Here's the drawing with two shaded views (mm, measured from the low corner). I have some questions. A direction names the side the tool comes from. Round coordinates to 2 decimals unless told otherwise and drop trailing zeros. Order: outer loops, then holes, each group sorted by start corner. A loop starts at its lowest first (then second) coordinate and runs counter-clockwise, first axis right, second up. Notation, with made-up numbers: (57, 20.5) - (102, 20.5) arc R6 cw to (102, 24.5) - close; hole circle Ø3 at (51, -19.5). An arc over 180 degrees is marked (long way). One line per item, written item: value.
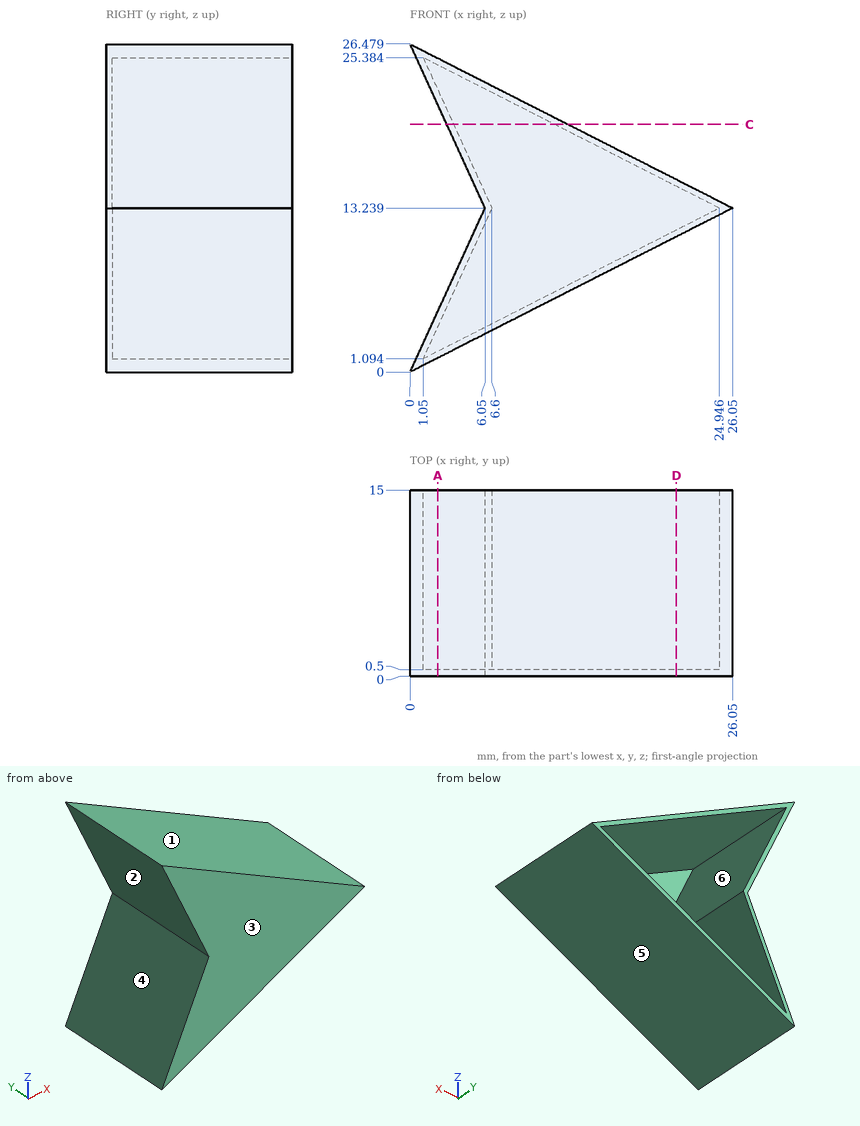
Q1. We'd pull the mould along Z, two halves only. Please class the marked faces 1, 2 and 3: released by +Z, released by -Z, zero draft, split by the parting line, or undercut.
Results list:
face 1: released by +Z
face 2: undercut
face 3: zero draft
Q2. If we section it at C-C, the plane z = 20: Please give me the cut outline in (x, y).
Results list:
outline: (2.96, 0) - (12.75, 0) - (12.75, 15) - (11.64, 15) - (11.64, 0.5) - (3.51, 0.5) - (3.51, 15) - (2.96, 15) - close
Q3. Will these pins go through, and if not, where does the flat tip stop? pin 1 (2 mm diameter, centred on y = 7, z = 17.5, fed in from -X) (1 decimal); pin 2 (5 mm diameter, centred on x = 7.5, y = 9, fed in from -Z); pin 3 (5 mm diameter, centred on y = 12, z = 22.5, fed in from -X) (1 decimal); pin 4 (3 mm diameter, centred on x = 16.5, z = 21, fed in from +Y).
Results list:
pin 1: x = 3.6
pin 2: z = 2.54
pin 3: x = 0.7
pin 4: through
Q4. If I drill on line 1 along Z through (x, y) = (7.75, 7.5); line 2 along X through (y, z) = (6.5, 13.75) (1 decimal); line 3 along Z through (x, y) = (16.25, 14), over which ranges is the centre line in solid material (lowest first)?
Results list:
line 1: 3.94 to 4.5, 21.98 to 22.54
line 2: 5.8 to 6.4, 23.9 to 25
line 3: 8.26 to 8.82, 17.66 to 18.22
Q5. Which directions (+Z, -Z, +X, -X, +Y, -Y) give clear straight access to the entire face, cutting with the end or side of a thin tool? Please do the marked faces 4, 5 and 6.
Results list:
face 4: -X, +Y, -Y
face 5: -Z, +X, +Y, -Y
face 6: +Y
Q6. If we section it at A-A, the plane x = 2.25: Please give me the cut outline in (y, z) (1 decimal).
Results list:
outline: (0, 1.1) - (15, 1.1) - (15, 1.7) - (0.5, 1.7) - (0.5, 3.7) - (15, 3.7) - (15, 4.9) - (0, 4.9) - close; (0, 21.6) - (15, 21.6) - (15, 22.8) - (0.5, 22.8) - (0.5, 24.8) - (15, 24.8) - (15, 25.3) - (0, 25.3) - close
Q7. If we section it at D-D, the plane x = 21.5: Please give me the cut outline in (y, z).
Results list:
outline: (0, 10.93) - (15, 10.93) - (15, 11.49) - (0.5, 11.49) - (0.5, 14.99) - (15, 14.99) - (15, 15.55) - (0, 15.55) - close
